For this review, take the finished solid that the model builds, in its own axes (mm). Face numbers are marked on the shaded views. A direction names the side the tool comes from. Coordinates: 2 decimals unless noted, no trailing zeros. Loops run counter-clockwise (first coordinate to the right, second up) from the corner with the lowest first, then second, coordinate; pieces in that order, holes last. Notation, with made-up numbers: M -1.75,61.5 L 22.25,61.5 A25 ccw 22.25,81.5 Z; hole C -12.5,-3.75 d4. An arc over 180 degrees is marked long. Answer as a JSON object with one key per item and string values. Group by question number.
Item 1: Wall thickness on L1, parallel to Z at x = 5, y = 6.75; L2, parallel to Y at x = 3, z = -5.75: over which ranges is each line inside the solid? List them lowest first. Write a range as from..to.
Item 2: Mouldability with a two-part tool opening along X and no side actions: class the marked faces 3, 4, 5 and 6 as +X half, -X half, draft (parallel to the pull), parting line (faces both ways), or undercut.
Item 3: Add section C-C (y = 1.75). State the section outline as (x, z) points, then the cut area to 3 significant figures.
Item 4: Tool access review of the marked faces 1 and 2: name each direction out of +Z, -Z, +X, -X, +Y, -Y from which nothing blocks a thin tool from reaching the whole face with its end or side.
Item 5: Add section D-D (z = -2.75). State the section outline as (x, y) points.
Item 6: Add section B-B (x = -8). State the section outline as (y, z) points.
Item 7: Add section A-A (y = 6.5). State the section outline as (x, z) points.
Item 8: Insertion check: pin 1 (1 mm diameter, centred on y = 5.5, z = 10, fed in from -X); pin 2 (8 mm diameter, centred on x = -3, z = -1.5, fed in from +Y). Each pin has a flat end and moves straight along its axis. Give the tip position at first contact, or say it passes through.
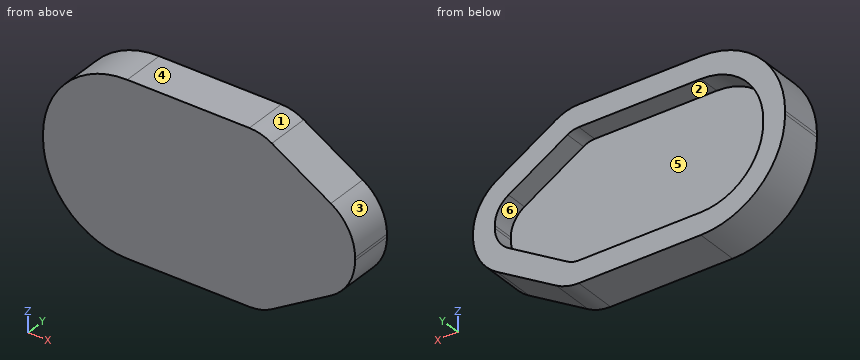
from build123d import *

# Parameters (mm, degrees)
SKETCH1_W           = 50
SKETCH1_H           = 27.5
BOSS_EXTRUDE1_DEPTH = 7
FILLET1_R           = 13.5
CUT_EXTRUDE1_REACH  = 31.378
FILLET2_R           = 8
FILLET3_R           = 7
SHELL1_T            = -3.5


with BuildPart() as part:
    # Sketch1 → Boss-Extrude1 (new body)
    with BuildSketch(Plane(origin=(0, 0, 0), x_dir=(1, 0, 0), z_dir=(0, 1, 0))):
        Rectangle(SKETCH1_W, SKETCH1_H)
    extrude(amount=BOSS_EXTRUDE1_DEPTH)

    # Fillet1
    fillet1_edges = [part.edges().sort_by_distance(p)[0] for p in [
        (-25, 3.5, 13.75),
        (-25, 3.5, -13.75),
    ]]
    fillet(fillet1_edges, radius=FILLET1_R)

    # Sketch3 → Cut-Extrude1 (cut, up to next)
    with BuildSketch(Plane(origin=(0, 7, 0), x_dir=(1, 0, 0), z_dir=(0, 1, 0)), mode=Mode.PRIVATE) as cut_extrude1_sk1:
        Polygon((10, 13.75), (25, 4.75), (25, 13.75), align=None)
    cut_extrude1_tool1 = extrude(cut_extrude1_sk1.sketch, amount=-CUT_EXTRUDE1_REACH, mode=Mode.PRIVATE) & part.part
    # Sketch3 → Cut-Extrude1 (cut, up to next)
    with BuildSketch(Plane(origin=(0, 7, 0), x_dir=(1, 0, 0), z_dir=(0, 1, 0)), mode=Mode.PRIVATE) as cut_extrude1_sk2:
        Polygon((25, -13.75), (10, -13.75), (25, -4.75), align=None)
    cut_extrude1_tool2 = extrude(cut_extrude1_sk2.sketch, amount=-CUT_EXTRUDE1_REACH, mode=Mode.PRIVATE) & part.part
    add(cut_extrude1_tool1.solids().sort_by_distance((20, 7, -10.75))[0], mode=Mode.SUBTRACT)
    add(cut_extrude1_tool2.solids().sort_by_distance((20, 7, 10.75))[0], mode=Mode.SUBTRACT)

    # Fillet2
    fillet2_edges = [part.edges().sort_by_distance(p)[0] for p in [
        (25, 3.5, -4.75),
        (25, 3.5, 4.75),
    ]]
    fillet(fillet2_edges, radius=FILLET2_R)

    # Fillet3
    fillet3_edges = [part.edges().sort_by_distance(p)[0] for p in [
        (10, 3.5, -13.75),
        (10, 3.5, 13.75),
    ]]
    fillet(fillet3_edges, radius=FILLET3_R)

    # Shell1
    shell1_openings = [part.faces().sort_by_distance(p)[0] for p in [
        (-0.99153661, 7, 0),
    ]]
    offset(amount=SHELL1_T, openings=shell1_openings, kind=Kind.INTERSECTION)


solid = part.part
From the geometry:
{
 "1": {"L1": "z = -13.75..-10.25, 10.25..13.75", "L2": "y = 0..3.5"},
 "2": {"face 3": "+X half", "face 4": "draft", "face 5": "undercut", "face 6": "undercut"},
 "3": {"outline": "M -25,-0.25 A13.5 ccw -11.5,-13.75 L 8.06,-13.75 A7 ccw 11.66,-12.75 L 21.12,-7.08 A8 ccw 25,-0.22 L 25,0.22 A8 ccw 21.12,7.08 L 11.66,12.75 A7 ccw 8.06,13.75 L -11.5,13.75 A13.5 ccw -25,0.25 Z", "area": "1,150 mm²"},
 "4": {"face 1": "+Z, +X, +Y, -Y", "face 2": "+Y"},
 "5": {"outline": "M -24.77,0 L 24.59,0 L 24.59,7 L 20.72,7 L 20.72,3.5 L -21.18,3.5 L -21.18,7 L -24.77,7 Z"},
 "6": {"outline": "M 0,-13.75 L 7,-13.75 L 7,-10.25 L 3.5,-10.25 L 3.5,10.25 L 7,10.25 L 7,13.75 L 0,13.75 Z"},
 "7": {"outline": "M -25,-0.25 A13.5 ccw -11.5,-13.75 L 8.06,-13.75 A7 ccw 11.66,-12.75 L 21.12,-7.08 A8 ccw 25,-0.22 L 25,0.22 A8 ccw 21.12,7.08 L 11.66,12.75 A7 ccw 8.06,13.75 L -11.5,13.75 A13.5 ccw -25,0.25 Z; hole M -21.5,-0.25 A10 ccw -11.5,-10.25 L 8.06,-10.25 A3.5 ccw 9.86,-9.75 L 19.32,-4.08 A4.5 ccw 21.5,-0.22 L 21.5,0.22 A4.5 ccw 19.32,4.08 L 9.86,9.75 A3.5 ccw 8.06,10.25 L -11.5,10.25 A10 ccw -21.5,0.25 Z"},
 "8": {"pin 1": "stops at x = -21.33", "pin 2": "stops at y = 3.5"}
}
